```python
from build123d import *

# Parameters (mm, degrees)
SKETCH1_W                = 200
SKETCH1_H                = 200
BOSS_EXTRUDE1_DEPTH      = 30
SKETCH4_W                = 175
SKETCH4_H                = 175
CUT_EXTRUDE1_DEPTH       = 30
SKETCH7_R                = 4
CUT_EXTRUDE2_DEPTH       = 210
SKETCH10_W               = 6.040230253
SKETCH10_H               = 30
BOSS_EXTRUDE2_DEPTH      = 20
SKETCH11_W               = 10
SKETCH11_H               = 30
BOSS_EXTRUDE3_DEPTH      = 20
CUT_EXTRUDE3_START       = -231
SKETCH12_R               = 4
CUT_EXTRUDE3_DEPTH       = 231
SKETCH13_R               = 4
CUT_EXTRUDE5_DEPTH       = 231
SKETCH14_R               = 4
CUT_EXTRUDE6_DEPTH       = 250.5
SKETCH15_R               = 30
SKETCH15_R_2             = 22
BOSS_EXTRUDE5_DEPTH      = 201
SKETCH17_R               = 22
CUT_EXTRUDE7_DEPTH       = 201
SKETCH21_W               = 9.5
SKETCH21_H               = 28.855904386
BOSS_EXTRUDE6_DEPTH      = 26
SKETCH22_W               = 9.5
SKETCH22_H               = 6.040230253
CUT_EXTRUDE10_DEPTH      = 49
SKETCH23_W               = 10.008922512
SKETCH23_H               = 28.855904386
BOSS_EXTRUDE7_DEPTH      = 21
SKETCH24_W               = 9.5
SKETCH24_H               = 1.144095614
CUT_EXTRUDE11_DEPTH      = 27
SKETCH26_W               = 0.50137975
SKETCH26_H               = 20.893624798
CUT_EXTRUDE12_DEPTH      = 35
SKETCH27_R               = 49.192783102
CUT_EXTRUDE13_DEPTH      = 175
SKETCH28_R               = 41.209023923
CUT_EXTRUDE14_DEPTH      = 175
SKETCH31_R               = 25.671187695
CUT_EXTRUDE15_DEPTH      = 175
CUT_EXTRUDE16_DEPTH      = 246.814971066
CUT_EXTRUDE16_DEPTH_BACK = 220


with BuildPart() as part:
    # Sketch1 → Boss-Extrude1 (new body)
    with BuildSketch(Plane(origin=(0, 0, 0), x_dir=(1, 0, 0), z_dir=(0, 1, 0))):
        Rectangle(SKETCH1_W, SKETCH1_H)
    extrude(amount=BOSS_EXTRUDE1_DEPTH)

    # Sketch4 → Cut-Extrude1 (cut)
    with BuildSketch(Plane(origin=(0, 30, 0), x_dir=(1, 0, 0), z_dir=(0, 1, 0))):
        Rectangle(SKETCH4_W, SKETCH4_H)
    extrude(amount=-CUT_EXTRUDE1_DEPTH, mode=Mode.SUBTRACT)

    # Sketch7 → Cut-Extrude2 (cut)
    with BuildSketch(Plane.ZY.offset(100)):
        with Locations((0, 15)):
            Circle(SKETCH7_R)
    extrude(amount=-CUT_EXTRUDE2_DEPTH, mode=Mode.SUBTRACT)

    # Sketch10 → Boss-Extrude2 (add)
    with BuildSketch(Plane.ZY.offset(100)):
        with Locations((-11.64671233, 15)):
            Rectangle(SKETCH10_W, SKETCH10_H)
    extrude(amount=BOSS_EXTRUDE2_DEPTH)

    # Sketch11 → Boss-Extrude3 (add)
    with BuildSketch(Plane.XY.offset(-8.626597203)):
        with Locations((-115, 15)):
            Rectangle(SKETCH11_W, SKETCH11_H)
    extrude(amount=BOSS_EXTRUDE3_DEPTH)

    # Sketch12 → Cut-Extrude3 (cut)
    with BuildSketch(Plane(origin=(100, 0, 0), x_dir=(0, 0, -1), z_dir=(1, 0, 0)).offset(CUT_EXTRUDE3_START)):
        with Locations(Location((0, 15, 0), (0, 0, 180))):
            Circle(SKETCH12_R)
    extrude(amount=CUT_EXTRUDE3_DEPTH, mode=Mode.SUBTRACT)

    # Sketch13 → Cut-Extrude5 (cut)
    with BuildSketch(Plane(origin=(0, 30, 0), x_dir=(1, 0, 0), z_dir=(0, 1, 0))):
        with Locations(Location((-93.69452155, -93.045501349, 0), (0, 0, 270))):
            Circle(SKETCH13_R)
    extrude(amount=-CUT_EXTRUDE5_DEPTH, mode=Mode.SUBTRACT)

    # Sketch14 → Cut-Extrude6 (cut)
    with BuildSketch(Plane.XY.offset(100)):
        with Locations((0, 13.614739596)):
            Circle(SKETCH14_R)
    extrude(amount=-CUT_EXTRUDE6_DEPTH, mode=Mode.SUBTRACT)

    # Sketch15 → Boss-Extrude5 (add)
    with BuildSketch(Plane(origin=(100, 0, 0), x_dir=(0, 0, -1), z_dir=(1, 0, 0))):
        with Locations((0, 15)):
            Circle(SKETCH15_R)
        with Locations((0, 15)):
            Circle(SKETCH15_R_2, mode=Mode.SUBTRACT)
    extrude(amount=-BOSS_EXTRUDE5_DEPTH)

    # Sketch17 → Cut-Extrude7 (cut)
    with BuildSketch(Plane(origin=(100, 0, 0), x_dir=(0, 0, -1), z_dir=(1, 0, 0))):
        with Locations((0.074377339, 15.100772812)):
            Circle(SKETCH17_R)
    extrude(amount=-CUT_EXTRUDE7_DEPTH, mode=Mode.SUBTRACT)


with BuildPart() as cut_extrude7_piece_1:
    # of the separate pieces the step leaves, piece 1, a body of its own (cut_extrude7_pieces)
    add(part.part.solids().sort_by_distance((-100, 0, -100))[0])



with BuildPart() as cut_extrude7_piece_2:
    # of the separate pieces the step leaves, piece 2, a body of its own (cut_extrude7_pieces)
    add(part.part.solids().sort_by_distance((-101, 0, -14.666827456))[0])

    # Sketch21 → Boss-Extrude6 (add)
    with BuildSketch(Plane(origin=(0, 0, -14.666827456), x_dir=(-1, 0, 0), z_dir=(0, 0, -1))):
        with Locations((115.25, 15.572047807)):
            Rectangle(SKETCH21_W, SKETCH21_H)
    extrude(amount=BOSS_EXTRUDE6_DEPTH)

    # Sketch22 → Cut-Extrude10 (cut)
    with BuildSketch(Plane(origin=(0, 30, 0), x_dir=(1, 0, 0), z_dir=(0, 1, 0))):
        with Locations((-105.75, 11.64671233)):
            Rectangle(SKETCH22_W, SKETCH22_H)
    extrude(amount=-CUT_EXTRUDE10_DEPTH, mode=Mode.SUBTRACT)


with BuildPart() as cut_extrude7_piece_1_1:
    add(cut_extrude7_piece_1.part)

    add(cut_extrude7_piece_2.part)  # Boss-Extrude7 merges Cut-Extrude7 piece 2
    # Sketch23 → Boss-Extrude7 (add)
    with BuildSketch(Plane(origin=(-110.5, 0, 0), x_dir=(0, 0, -1), z_dir=(1, 0, 0))):
        with Locations((35.6623662, 15.572047807)):
            Rectangle(SKETCH23_W, SKETCH23_H)
    extrude(amount=BOSS_EXTRUDE7_DEPTH)

    # Sketch24 → Cut-Extrude11 (cut)
    with BuildSketch(Plane(origin=(0, 0, -14.666827456), x_dir=(-1, 0, 0), z_dir=(0, 0, -1))):
        with Locations((115.25, 0.572047807)):
            Rectangle(SKETCH24_W, SKETCH24_H)
    extrude(amount=-CUT_EXTRUDE11_DEPTH, mode=Mode.SUBTRACT)

    # Sketch26 → Cut-Extrude12 (cut)
    with BuildSketch(Plane.XZ):
        with Locations((-110.249310125, 1.820215196)):
            Rectangle(SKETCH26_W, SKETCH26_H)
    extrude(amount=-CUT_EXTRUDE12_DEPTH, mode=Mode.SUBTRACT)

    # Sketch27 → Cut-Extrude13 (cut)
    with BuildSketch(Plane(origin=(-87.5, 0, 0), x_dir=(0, 0, -1), z_dir=(1, 0, 0))):
        with Locations((-31.916352411, 15.376133278)):
            Circle(SKETCH27_R)
    extrude(amount=CUT_EXTRUDE13_DEPTH, mode=Mode.SUBTRACT)

    # Sketch28 → Cut-Extrude14 (cut)
    with BuildSketch(Plane(origin=(-87.5, 0, 0), x_dir=(0, 0, -1), z_dir=(1, 0, 0))):
        with Locations((37.762434774, 15.494435184)):
            Circle(SKETCH28_R)
    extrude(amount=CUT_EXTRUDE14_DEPTH, mode=Mode.SUBTRACT)

    # Sketch31 → Cut-Extrude15 (cut)
    with BuildSketch(Plane(origin=(-87.5, 0, 0), x_dir=(0, 0, -1), z_dir=(1, 0, 0))):
        with Locations((-2.206126603, -10.850671417)):
            Circle(SKETCH31_R)
    extrude(amount=CUT_EXTRUDE15_DEPTH, mode=Mode.SUBTRACT)

    # Sketch32 → Cut-Extrude16 (cut, two sides: drawn at the far end of the back side and taken through both)
    with BuildSketch(Plane(origin=(100, 0, 0), x_dir=(0, 0, -1), z_dir=(1, 0, 0)).offset(-CUT_EXTRUDE16_DEPTH_BACK)):
        with BuildLine():
            Line((112.795739645, 270.367951942), (-25.980762114, 30))
            ThreePointArc((-25.980762114, 30), (-30, 15), (-25.980762114, 0))
            Line((-25.980762114, 0), (112.795739645, -240.367951942))
            Line((112.795739645, -240.367951942), (667.901746678, -240.367951942))
            Line((667.901746678, -240.367951942), (667.901746678, 270.367951942))
            Line((667.901746678, 270.367951942), (112.795739645, 270.367951942))
        make_face()
    extrude(amount=CUT_EXTRUDE16_DEPTH + CUT_EXTRUDE16_DEPTH_BACK, mode=Mode.SUBTRACT)


solid = cut_extrude7_piece_1_1.part
```
Here's how the part is built. I have some questions about the finished solid (model axes, mm). A direction names the side the tool comes from. Round coordinates to 2 decimals unless told otherwise and drop trailing zeros. Order: outer loops, then holes, each group sorted by start corner. A loop starts at its lowest first (then second) coordinate and runs counter-clockwise, first axis right, second up. Notation, with made-up numbers: M 34,19 L 51,19 A31 ccw 51,43 Z; hole C -12.5,82 d7. An arc over 180 degrees is marked long. Use CSV: the item, a comma, the result in double quotes.
1) I want a section at B-B (x = 0). List the corners of the cut face in (y, z) for me.
Taken from the geometry:
outline,"M 0,87.5 L 9.61,87.5 L 9.61,100 L 0,100 Z; M 17.61,87.5 L 30,87.5 L 30,100 L 17.61,100 Z"
2) I want a section at A-A (z = 83). List the corners of the cut face in (x, y) for me.
Taken from the geometry:
outline,"M -100,0 L -87.5,0 L -87.5,30 L -100,30 Z; M 87.5,0 L 100,0 L 100,30 L 87.5,30 Z"
3) I want a section at C-C (y = 4). List the corners of the cut face in (x, z) for me, then the cut area to 3 significant figures.
Taken from the geometry:
outline,"M -100,27.91 L -87.5,27.91 L -87.5,87.5 L 87.5,87.5 L 87.5,27.91 L 100,27.91 L 100,100 L -100,100 Z; hole C -93.69,93.05 d8"
area,"3,940 mm^2"
4) I need wall thicknesses on line 1 along X through (y, z) = (11, 32); line 2 along Y through (x, z) = (0, 90.5); line 3 along Z through (x, y) = (40.5, 7). Which ranges of each line are inside material? Lowest first, please. Write a range as [from, to].
Taken from the geometry:
line 1,"[-100, -87.5], [87.5, 100]"
line 2,"[0, 9.61], [17.61, 30]"
line 3,"[87.5, 100]"
5) On a 3-axis mill with a long thin cutter (end or side, diameter ignored), from which of +Z, -Z, +X, -X, +Y, -Y can I reach the whole of each face in a straight line? I mean faces 1 (the flat face through (87.5, 15, 57)), 2 (the flat face through (0, 0, 90)). Say none if no direction works.
Taken from the geometry:
face 1,"-Z, +Y, -Y"
face 2,"+Z, -Z, +X, -X, -Y"
6) If we mould it in two halves opening along X, with no side actions, what happens to faces 3 (the cylindrical face through (-97.6, 15.21, 92.18)), 4 (the flat face through (0, 30, 90)), 5 (the flat face through (-100, 15, 64))? For each: pulls with the +X half, pulls with the -X half, needs draft (parallel to the pull), parting line crosses it, or undercut.
Taken from the geometry:
face 3,"undercut"
face 4,"needs draft"
face 5,"pulls with the -X half"
7) I'm going to push flat-ended pins straight in: P1, Ø2, axis at x = -31.5, y = 23, coming from the -Z side; P2, Ø7, axis at x = -93.69, z = 93.05, coming from the -Y side. Where does each tip first touch, or does it pass through?
Taken from the geometry:
P1,"z = 87.5"
P2,"through"
